```python
from build123d import *

# Parameters (mm, degrees)
SKETCH1_W             = 172.72
SKETCH1_H             = 76.2
BOSS_EXTRUDE1_DEPTH   = 5.85
SKETCH2_W             = 5.85
SKETCH2_H             = 25.4
SKETCH2_W_2           = 41.691074393
SKETCH2_H_2           = 8.720383817
SKETCH2_W_3           = 43.92952134
SKETCH2_W_4           = 45.443124842
SKETCH2_H_3           = 50
CUT_EXTRUDE1_DEPTH    = 10
SKETCH3_W             = 29.139699911
SKETCH3_H             = 25.4
BOSS_EXTRUDE2_DEPTH   = 5.85
SKETCH3_W_2           = 38.893015708
BOSS_EXTRUDE2_2_DEPTH = 5.85
SKETCH3_W_3           = 19.066688648
BOSS_EXTRUDE2_3_DEPTH = 5.85
SKETCH4_W             = 9.977498033
SKETCH4_H             = 25.4
SKETCH4_W_2           = 10.229966749
SKETCH4_W_3           = 9.637990001
CUT_EXTRUDE2_DEPTH    = 10
CAVITY1_START         = -38.1
CAVITY1_OUTLINE_W     = 12.130208491
CAVITY1_OUTLINE_H     = 5.85
CAVITY1_OUTLINE_W_2   = 57.573333333
CAVITY1_DEPTH         = 11.7
FILLET2_R             = 20


# Read off the part's stored shape, not the designer's step: Cavity1
with BuildPart() as part:
    # Sketch1 → Boss-Extrude1 (new body)
    with BuildSketch(Plane(origin=(0, 0, 0), x_dir=(1, 0, 0), z_dir=(0, 1, 0))):
        Rectangle(SKETCH1_W, SKETCH1_H)
    extrude(amount=BOSS_EXTRUDE1_DEPTH)

    # Sketch2 → Cut-Extrude1 (cut)
    with BuildSketch(Plane(origin=(0, 5.85, 0), x_dir=(1, 0, 0), z_dir=(0, 1, 0))):
        with Locations((-83.435, 0)):
            Rectangle(SKETCH2_W, SKETCH2_H)
        with Locations((-46.447774155, -33.739808092)):
            Rectangle(SKETCH2_W_2, SKETCH2_H_2)
        with Locations((35.255539419, -33.739808092)):
            Rectangle(SKETCH2_W_3, SKETCH2_H_2)
        with Locations((63.638437579, 13.1)):
            Rectangle(SKETCH2_W_4, SKETCH2_H_3)
    extrude(amount=-CUT_EXTRUDE1_DEPTH, mode=Mode.SUBTRACT)


with BuildPart() as body_2:
    # Sketch3 → Boss-Extrude2 (new body)
    with BuildSketch(Plane(origin=(0, 5.85, 0), x_dir=(-1, 0, 0), z_dir=(0, 1, 0))):
        with Locations((-71.790150044, 50.8)):
            Rectangle(SKETCH3_W, SKETCH3_H)
    extrude(amount=-BOSS_EXTRUDE2_DEPTH)


with BuildPart() as body_3:
    # Sketch3 → Boss-Extrude2 2 (new body)
    with BuildSketch(Plane(origin=(0, 5.85, 0), x_dir=(-1, 0, 0), z_dir=(0, 1, 0))):
        with Locations((6.155729105, 50.8)):
            Rectangle(SKETCH3_W_2, SKETCH3_H)
    extrude(amount=-BOSS_EXTRUDE2_2_DEPTH)


with BuildPart() as body_4:
    # Sketch3 → Boss-Extrude2 3 (new body)
    with BuildSketch(Plane(origin=(0, 5.85, 0), x_dir=(-1, 0, 0), z_dir=(0, 1, 0))):
        with Locations((76.826655676, 50.8)):
            Rectangle(SKETCH3_W_3, SKETCH3_H)
    extrude(amount=-BOSS_EXTRUDE2_3_DEPTH)


with BuildPart() as part_1:
    add(part.part)

    # Combine1: union body 4, body 3, body 2
    add(body_4.part)
    add(body_3.part)
    add(body_2.part)

    # Sketch4 → Cut-Extrude2 (cut)
    with BuildSketch(Plane(origin=(0, 5.85, 0), x_dir=(1, 0, 0), z_dir=(0, 1, 0))):
        with Locations((-20.613487943, -50.8)):
            Rectangle(SKETCH4_W, SKETCH4_H)
        with Locations((8.175795375, -50.8)):
            Rectangle(SKETCH4_W_2, SKETCH4_H)
        with Locations((62.03929509, -50.8)):
            Rectangle(SKETCH4_W_3, SKETCH4_H)
    extrude(amount=-CUT_EXTRUDE2_DEPTH, mode=Mode.SUBTRACT)

    # Cavity1 outline → Cavity1 (cut)
    with BuildSketch(Plane.XY.offset(CAVITY1_START)):
        with Locations((34.851770913, 2.925)):
            Rectangle(CAVITY1_OUTLINE_W, CAVITY1_OUTLINE_H)
        with Locations((-57.573333334, 2.925)):
            Rectangle(CAVITY1_OUTLINE_W_2, CAVITY1_OUTLINE_H)
    extrude(amount=CAVITY1_DEPTH, mode=Mode.SUBTRACT)

    # Fillet2
    fillet2_edges = [part_1.edges().sort_by_distance(p)[0] for p in [
        (86.36, 2.925, 11.9),
    ]]
    fillet(fillet2_edges, radius=FILLET2_R)


solid = part_1.part
```
The model under review builds one solid part; all positions refer to its coordinate system, in mm. A direction names the side the tool comes from. Round coordinates to 2 decimals unless told otherwise and drop trailing zeros. Loops run counter-clockwise (first coordinate to the right, second up) from the corner with the lowest first, then second, coordinate; pieces in that order, holes last. Notation, with made-up numbers: (-14, 19.25) -> (-4, 19.25) arc R22 ccw to (-4, 56.25) -> close; hole circle Ø1 at (-21.5, 89). An arc over 180 degrees is marked (long way). Answer as a JSON object with one key per item and string values. Group by question number.
1) We need section D-D on z = 34.5. Write out the cut boundary in (x, y).
2) Mouldability with a two-part tool opening along X and no side actions: class faces 1 (the face through (-80.51, 3, 0)), 2 (the face through (35, 3, -26.4)), 3 (the face through (3.061, 3, 51)) as released by +X, released by -X, zero draft, split by the parting line, or undercut.
3) For faces 4 (the face through (-21, 3, 38.1)), 5 (the face through (77, 3, 63.5)), 6 (the face through (-58, 3, -26.4)), 7 (the face through (-83, 3, 12.7)), list the 3-axis set-ups (+Z, -Z, +X, -X, +Y, -Y) from which the entire face can be reached by the end or side of a thin tool; tool diameter is ignored.
4) For line 1 (X direction, y = 4.8, z = 35); line 2 (X direction, y = 1.75, z = 39); line 3 (X direction, y = 0.75, z = -22.5), list the stretches that pass through material, from the lowest coordinate up. Write a range as [from, to].
5) For pin 1 Ø1.8 at (y, z) = (3.5, -31) entering from +X; pin 2 Ø1.8 at (x, y) = (-22.5, 3) entering from +Z; pin 3 Ø1.8 at (y, z) = (1.5, -32) entering from -X; pin 4 Ø1.8 at (y, z) = (2, 31.5) entering from +X, all flat-tipped, find the tip position at first contact; note any pin that passes through.
6) We need section A-A on z = 54. Write out the cut boundary in (x, y).
7) We need section C-C on x = -53. Write out the cut boundary in (y, z), then the cut area to 3 significant figures.
Result set:
{
 "1": {"outline": "(-86.36, 0) -> (-67.29, 0) -> (-67.29, 5.85) -> (-86.36, 5.85) -> close; (-25.6, 0) -> (13.29, 0) -> (13.29, 5.85) -> (-25.6, 5.85) -> close; (57.22, 0) -> (86.36, 0) -> (86.36, 5.85) -> (57.22, 5.85) -> close"},
 "2": {"face 1": "released by -X", "face 2": "zero draft", "face 3": "undercut"},
 "3": {"face 4": "+Z, +Y, -Y", "face 5": "+Z, +X, -X, +Y, -Y", "face 6": "-Z, -X, +Y, -Y", "face 7": "-X, +Y, -Y"},
 "4": {"line 1": "[-86.36, -67.29], [-25.6, 13.29], [57.22, 86.36]", "line 2": "[-86.36, -67.29], [-15.62, 3.06], [66.86, 86.36]", "line 3": "[-86.36, 40.92]"},
 "5": {"pin 1": "x = 28.79", "pin 2": "z = 38.1", "pin 3": "x = -28.79", "pin 4": "x = 86.36"},
 "6": {"outline": "(-86.36, 0) -> (-67.29, 0) -> (-67.29, 5.85) -> (-86.36, 5.85) -> close; (-15.62, 0) -> (3.06, 0) -> (3.06, 5.85) -> (-15.62, 5.85) -> close; (66.86, 0) -> (86.36, 0) -> (86.36, 5.85) -> (66.86, 5.85) -> close"},
 "7": {"outline": "(0, -26.4) -> (5.85, -26.4) -> (5.85, 29.38) -> (0, 29.38) -> close", "area": "326 mm²"}
}
